from build123d import *

# Parameters (mm, degrees)
PAD_DEPTH       = 6
POCKET_DEPTH    = 2.85
CHAMFER_SIZE    = 1.849
CHAMFER001_SIZE = 2


with BuildPart() as part:
    # Sketch → Pad (new body)
    with BuildSketch(Plane.XZ):
        with BuildLine():
            ThreePointArc((-9, -4.00004), (2e-05, -13.00004), (9, -4))
            Line((9, 7), (9, -4))
            Line((-9, 7), (9, 7))
            Line((-9, -4.00004), (-9, 7))
        make_face()
        with BuildLine():
            ThreePointArc((2.15, 0), (0, 2.15), (-2.15, 0))
            Line((-2.15, 0), (-2.15, -4.00004))
            ThreePointArc((-2.15, -4.00004), (0, -6.15004), (2.15, -4.00004))
            Line((2.15, 0), (2.15, -4.00004))
        make_face(mode=Mode.SUBTRACT)
    extrude(amount=PAD_DEPTH)

    # Sketch001 → Pocket (cut)
    with BuildSketch(Plane.XZ.offset(6)):
        with BuildLine():
            ThreePointArc((4, 0), (0, 4), (-4, 0))
            Line((-4, 0), (-4, -4.00004))
            ThreePointArc((-4, -4.00004), (0, -8.00004), (4, -4.00004))
            Line((4, 0), (4, -4.00004))
        make_face()
    extrude(amount=-POCKET_DEPTH, mode=Mode.SUBTRACT)

    # Chamfer
    chamfer_edges = [part.edges().sort_by_distance(p)[0] for p in [
        (-4, -3.15, -2.00002),
    ]]
    chamfer(chamfer_edges, length=CHAMFER_SIZE)

    # Chamfer001
    chamfer001_edges = [part.edges().sort_by_distance(p)[0] for p in [
        (-9, -6, 1.49998),
    ]]
    chamfer(chamfer001_edges, length=CHAMFER001_SIZE)


solid = part.part
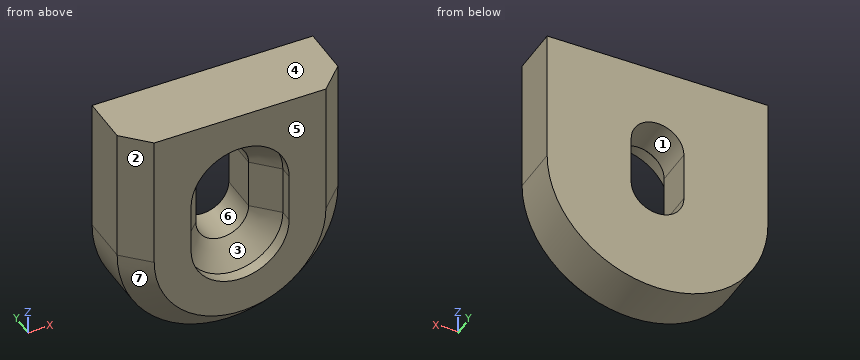
Source: CAD feature listing. Evaluate the final solid. Frame: model axes, mm. Face numbers are marked on the shaded views. A direction names the side the tool comes from. Round coordinates to 2 decimals unless told otherwise and drop trailing zeros. Loops run counter-clockwise (first coordinate to the right, second up) from the corner with the lowest first, then second, coordinate; pieces in that order, holes last.
Q1. Mould query, pull axis Z, two halves, no side actions, for the marked faces 4, 5, 6 and 7. Classes: pulls with the +Z half, pulls with the -Z half, needs draft (parallel to the pull), parting line crosses it, or undercut.
Q2. Section D-D, the plane z = 5.75. Return loops of the section in (x, y).
Q3. First-contact query: P1, Ø3.5, axis at x = 1, z = -1, coming from the -Y side; P2, Ø0.5, axis at y = -5.5, z = -1, coming from the -X side. Flat tips, straight axial feed; report the tip coordinate or a pass-through.
Q4. Ray query, line 1 (Z direction, x = 0, y = -2); line 2 (X direction, y = -1.75, z = -3.25); line 3 (Z direction, x = -1.75, y = -3.5). Return the intervals inside material, ascending.
Q5. Access query for the marked faces 1, 2 and 3. Directions: +Z, -Z, +X, -X, +Y, -Y. A direction counts if a zero-diameter tool reaches every point of the face in a straight line with its end or side. Return the directions, or none.
Q6. Section C-C, the plane y = -2.5. Return loops of the section in (x, z), plus the area to 3 significant figures.
Solutions:
1. face 4: pulls with the +Z half
1. face 5: needs draft
1. face 6: undercut
1. face 7: pulls with the -Z half
2. outline: (-9, -4) - (-7, -6) - (7, -6) - (9, -4) - (9, 0) - (-9, 0) - close
3. P1: stops at y = -3.75
3. P2: stops at x = -7.75
4. line 1: z = -13 to -6.15, 2.15 to 7
4. line 2: x = -9 to -2.15, 2.15 to 9
4. line 3: z = -12.83 to -5.79, 1.79 to 7
5. face 1: +Y, -Y
5. face 2: +Z, -Z, -X, -Y
5. face 3: -Y
6. outline: (-9, -4) arc R9 ccw to (9, -4) - (9, 7) - (-9, 7) - close; hole (-2.15, -4) arc R2.15 ccw to (2.15, -4) - (2.15, 0) arc R2.15 ccw to (-2.15, 0) - close
6. area: 294 mm2
